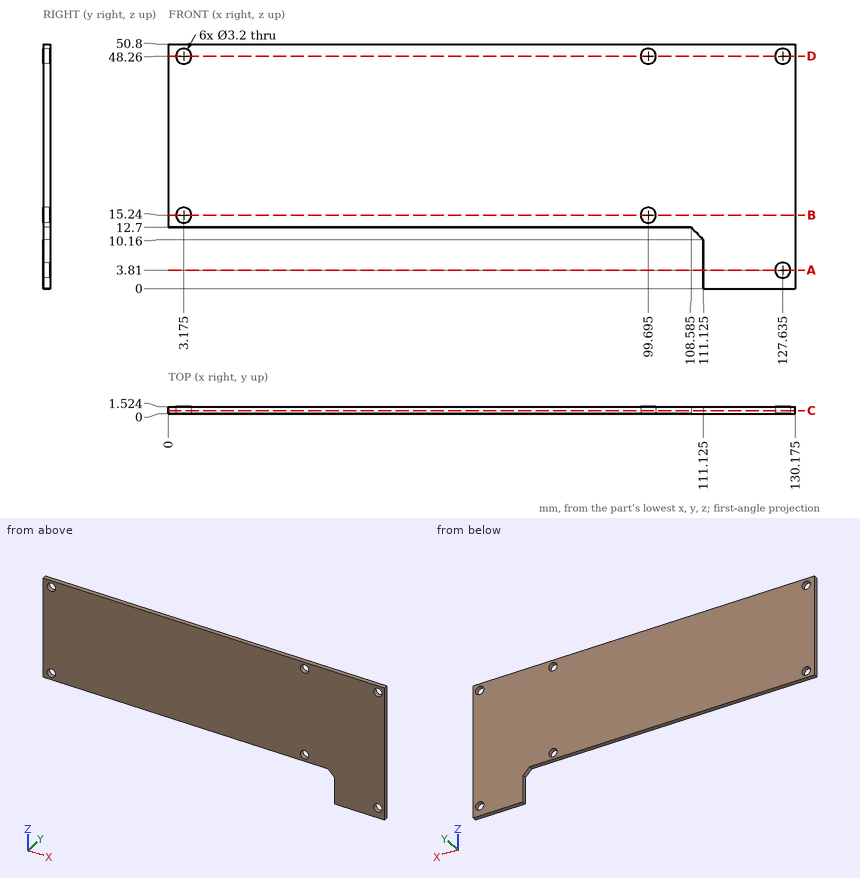
Geometry: see drawing. Coordinates: mm, zero at the bounding-box minimum. Give positions to 0.01 mm unless a question says otherwise; leave off trailing zeros. Loops run counter-clockwise (first coordinate to the right, second up) from the corner with the lowest first, then second, coordinate; pieces in that order, holes last. Notation, with made-up numbers: (79.25, -34.5) - (112.25, -34.5) arc R15 ccw to (112.25, -24.5) - close; hole circle Ø8 at (67.5, -7.75). An arc over 180 degrees is marked (long way). Use CSV: the item, a comma, the result in double quotes. Start each with the question number.
Item 1: Line query: line 1 (X direction, y = 0.7, z = 48) (3 decimals); line 2 (Z direction, x = 103, y = 1.4); line 3 (X direction, y = 0.55, z = 7) (3 decimals). Output: solid intervals per line, ascending.
Item 2: Contact query for a flat-ended pin moving along its axis: P1, Ø0.5, axis at x = 50.5, y = 1, coming from the -Z side. Output: stop coordinate, or through.
Item 3: Section A-A on z = 3.81. Return loops of the section in (x, y) (3 decimals), then the cut area to 3 significant figures.
Item 4: Section D-D on z = 48.26. Return loops of the section in (x, y) (3 decimals).
Item 5: Section C-C on y = 0.7. Return loops of the section in (x, z) (3 decimals), then the cut area to 3 significant figures.
Item 6: Section B-B on z = 15.24. Return loops of the section in (x, y) (3 decimals), then the cut area to 3 significant figures.
Ans:
1,line 1,"x = 0 to 1.596, 4.754 to 98.116, 101.274 to 126.056, 129.214 to 130.175"
1,line 2,"z = 12.7 to 50.8"
1,line 3,"x = 111.125 to 130.175"
2,P1,"stops at z = 12.7"
3,outline,"(111.125, 0) - (126.035, 0) - (126.035, 1.524) - (111.125, 1.524) - close; (129.235, 0) - (130.175, 0) - (130.175, 1.524) - (129.235, 1.524) - close"
3,area,"24.2 mm2"
4,outline,"(0, 0) - (1.575, 0) - (1.575, 1.524) - (0, 1.524) - close; (4.775, 0) - (98.095, 0) - (98.095, 1.524) - (4.775, 1.524) - close; (101.295, 0) - (126.035, 0) - (126.035, 1.524) - (101.295, 1.524) - close; (129.235, 0) - (130.175, 0) - (130.175, 1.524) - (129.235, 1.524) - close"
5,outline,"(0, 12.7) - (108.585, 12.7) - (111.125, 10.16) - (111.125, 0) - (130.175, 0) - (130.175, 50.8) - (0, 50.8) - close; hole circle Ø3.2 at (3.175, 15.24); hole circle Ø3.2 at (3.175, 48.26); hole circle Ø3.2 at (99.695, 15.24); hole circle Ø3.2 at (99.695, 48.26); hole circle Ø3.2 at (127.635, 3.81); hole circle Ø3.2 at (127.635, 48.26)"
5,area,"5,160 mm2"
6,outline,"(0, 0) - (1.575, 0) - (1.575, 1.524) - (0, 1.524) - close; (4.775, 0) - (98.095, 0) - (98.095, 1.524) - (4.775, 1.524) - close; (101.295, 0) - (130.175, 0) - (130.175, 1.524) - (101.295, 1.524) - close"
6,area,"189 mm2"
